Geometry check sheet. Reference: the model listing, model coordinates, mm. A direction names the side the tool comes from. Round coordinates to 2 decimals unless told otherwise and drop trailing zeros. Loops run counter-clockwise (first coordinate to the right, second up) from the corner with the lowest first, then second, coordinate; pieces in that order, holes last. Notation, with made-up numbers: M 66,-13.75 L 79,-13.75 A19 ccw 79,5.25 Z; hole C -8,3 d1. An arc over 180 degrees is marked long. Write item = value, one per line.
from build123d import *

# Parameters (mm, degrees)
SKETCH_R        = 10
PAD_DEPTH       = 35
SKETCH001_R     = 2.75
POCKET_DEPTH    = 35.001
SKETCH002_R     = 5
POCKET001_DEPTH = 10


with BuildPart() as part:
    # Sketch → Pad (new body)
    with BuildSketch(Plane.XY):
        Circle(SKETCH_R)
    extrude(amount=PAD_DEPTH)

    # Sketch001 (on Face3 of Pad) → Pocket (cut, through all)
    with BuildSketch(Plane.XY.offset(35)):
        Circle(SKETCH001_R)
    extrude(amount=-POCKET_DEPTH, mode=Mode.SUBTRACT)

    # Sketch002 (on Face3 of Pocket) → Pocket001 (cut)
    with BuildSketch(Plane.XY.offset(35)):
        Circle(SKETCH002_R)
    extrude(amount=-POCKET001_DEPTH, mode=Mode.SUBTRACT)


solid = part.part
(1) Release check for a two-part mould opening along X. For faces 3 (the flat face through (-5, -2, 35)), 4 (the cylindrical face through (-2.17, -9.76, 17.26)), 5 (the flat face through (2.2, -2.2, 25)) record: released by +X, released by -X, zero draft, split by the parting line, or undercut.
Result set:
face_3 = zero draft
face_4 = split by the parting line
face_5 = undercut
(2) Sectioned sample at A-A on x = 0. Record the cut outline in (y, z), then the cut area to 4 significant figures.
Result set:
outline = M -10,0 L -2.75,0 L -2.75,25 L -5,25 L -5,35 L -10,35 Z; M 2.75,0 L 10,0 L 10,35 L 5,35 L 5,25 L 2.75,25 Z
area = 462.5 mm2
(3) Sectioned sample at C-C on z = 30. Record the cut outline in (x, y).
Result set:
outline = C 0,0 d20; hole C 0,0 d10
(4) Tool access check on faces 1 (the flat face through (2.1, -2.1, 0)), 2 (the cylindrical face through (-1.08, -4.88, 30.07)). Record the directions out of +Z, -Z, +X, -X, +Y, -Y that give a thin tool (end or side, any length) a straight path to the whole face; none if there is none.
Result set:
face_1 = -Z, +X, -X, +Y, -Y
face_2 = +Z
(5) Material ranges on line 1 along Y through (x, z) = (0, 29); line 2 along Y through (x, z) = (0, 12); line 3 along X through (y, z) = (1.75, 21.5), recorded low to high. Write a range as from..to.
Result set:
line_1 = -10..-5, 5..10
line_2 = -10..-2.75, 2.75..10
line_3 = -9.85..-2.12, 2.12..9.85
(6) Depth check by flat-ended pin: pin 1 Ø5 at (x, y) = (4.5, -1.5) entering from -Z; pin 2 Ø6 at (x, z) = (-5, 27.5) entering from -Y; pin 3 Ø3 at (x, y) = (-2, -2) entering from +Z; pin 4 Ø1 at (x, z) = (-7.5, 12.5) entering from +Y. Enter the tip coordinate at first touch or a pass-through.
Result set:
pin_1 = 0
pin_2 = -9.8
pin_3 = 25
pin_4 = 7.14
(7) Sectioned sample at D-D on x = -3.25. Record the cut outline in (y, z), then the cut area to 3 significant figures.
Result set:
outline = M -9.46,0 L 9.46,0 L 9.46,35 L 3.8,35 L 3.8,25 L -3.8,25 L -3.8,35 L -9.46,35 Z
area = 586 mm2
